Autodesk Inventor part; units mm, degrees
ref_plane "YZ Plane" through (0, 0, 0) normal (1, 0, 0) x (0, 1, 0)
ref_plane "XZ Plane" through (0, 0, 0) normal (0, 1, 0) x (-1, 0, 0)
ref_plane "XY Plane" through (0, 0, 0) normal (0, 0, 1) x (1, 0, 0)
sketch "Skizze1" plane through (0, 0, 0) normal (0, 0, 1) x (1, 0, 0)
  line L0 (-71.4, 0) -> (71.4, 0)
  line L1 (0, -4.2) -> (0, 4.2)
  line L2 (-51, -3) -> (51, -3)
  line L3 (51, -3) -> (51, 3)
  line L4 (51, 3) -> (-51, 3)
  line L5 (-51, 3) -> (-51, -3)
  line L6 (-51, -3) -> (51, 3) construction
  line L7 (51, -3) -> (-51, 3) construction
  point P0 (0, 0)
  dimension "d0" = 102
  dimension "d1" = 6
extrude "Extrusion1" add sketch "Skizze1" against normal blind 348
sketch "Skizze2" plane through (-51, 3, 0) normal (0, 1, 0) x (1, 0, 0)
  line L0 (102, 0) -> (0, 0)
  line L1 (102, 0) -> (102, 348)
  line L2 (0, 348) -> (102, 348)
  line L3 (0, 0) -> (0, 348)
  line L4 (-20.4, 0) -> (122.4, 0)
  line L5 (51, 417.6) -> (51, -69.6)
  line L6 (0, 0) -> (102, 0)
  line L7 (0, 0) -> (6, 0)
  line L8 (6, 0) -> (6, 7)
  line L9 (6, 7) -> (0, 7)
  line L10 (0, 7) -> (0, 0)
  line L11 (102, 0) -> (96, 0)
  line L12 (96, 0) -> (96, 7)
  line L13 (96, 7) -> (102, 7)
  line L14 (102, 7) -> (102, 0)
  line L15 (102, 0) -> (102, 348)
  line L16 (102, 348) -> (96, 348)
  line L17 (96, 348) -> (96, 341)
  line L18 (96, 341) -> (102, 341)
  line L19 (102, 341) -> (102, 348)
  line L20 (102, 348) -> (0, 348)
  line L21 (0, 348) -> (6, 348)
  line L22 (6, 348) -> (6, 341)
  line L23 (6, 341) -> (0, 341)
  line L24 (0, 341) -> (0, 348)
  point P0 (51, 0)
  point P1 (0, 7)
  point P2 (6, 0)
  dimension "d4" = 6
  dimension "d5" = 7
  dimension "d6" = 6
  dimension "d7" = 7
  dimension "d8" = 6
extrude "Extrusion2" cut sketch "Skizze2" against normal blind 348 contours L0 L12 L13 L1 | L18 L17 L2 L1 | L0 L3 L9 L8 | L22 L23 L3 L2
sketch "Skizze3" plane through (51, 3, -7) normal (1, 0, 0) x (0, 0, -1)
  line L0 (334, -6) -> (334, 0)
  line L1 (0, 0) -> (334, 0)
  line L2 (0, 0) -> (0, -6)
  line L3 (0, -6) -> (334, -6)
  point P0 (-7, -3)
  point P1 (23.5, -3)
  point P2 (167, -3)
  point P3 (310.5, -3)
  dimension "d11" = 23.5
  dimension "d12" = 23.5
  dimension "d13" = 167
hole "Bohrung1" at (51, 0, -30.5) at (51, 0, -174) at (51, 0, -317.5) direction (-1, 0, 0) diameter 2.459 depth 8.8 tip angle 118
sketch "Skizze4" plane through (0, 0, 0) normal (0, 0, 1) x (1, 0, 0)
  line L0 (-45, 3) -> (-45, -3)
  line L1 (-45, -3) -> (45, -3)
  line L2 (45, -3) -> (45, 3)
  line L3 (45, 3) -> (-45, 3)
  line L4 (-71.4, 0) -> (71.4, 0)
  line L5 (0, -4.2) -> (0, 4.2)
  point P0 (0, 0)
  point P1 (0, 0)
hole "Bohrung2" at (0, 0, 0) direction (0, 0, -1) diameter 2.459 depth 17 tip angle 118
sketch "Skizze5" plane through (-51, 3, -341) normal (-1, 0, 0) x (0, 0, 1)
  line L0 (334, -6) -> (334, 0)
  line L1 (334, 0) -> (0, 0)
  line L2 (0, 0) -> (0, -6)
  line L3 (334, -6) -> (0, -6)
  circle A0 centre (310.5, -3) radius 1.2295
  circle A1 centre (167, -3) radius 1.2295
  circle A2 centre (23.5, -3) radius 1.2295
  line L4 (341, -7.2) -> (341, 1.2)
  line L5 (-76.6, -3) -> (410.6, -3)
  circle A3 centre (23.5, -3) radius 1.2295
  point P0 (341, -3)
hole "Bohrung3" at (-51, 0, -317.5) at (-51, 0, -174) at (-51, 0, -30.5) direction (1, 0, 0) diameter 2.459 depth 17 tip angle 118
properties part number "I Bodenplatte" material "PVC, hart"
Verification items for the finished model (mm, model axes). A direction names the side the tool comes from. Give positions to 0.01 mm unless a question says otherwise; leave off trailing zeros.
(1) Gauge pin test, flat ends, axial feed: pin 1 (2 mm diameter, centred on y = 0, z = -30.5, fed in from +X); pin 2 (1.8 mm diameter, centred on x = 47, y = -0.5, fed in from +Z); pin 3 (1.8 mm diameter, centred on x = -47, y = 0.5, fed in from -Z). Record the tip position at first contact, or that the pin passes through.
(2) Access from +Z, -Z, +X, -X, +Y, -Y to the whole of each face (thin tool, end or side, straight path). Record for faces 1 (the face through (-48, 0, -341)), 2 (the face through (48, 0, -341)), 3 (the face through (51, 0, -172)), 4 (the face through (-45, 0, -3)), 5 (the face through (45, 0, -3)).
(3) Material ranges on line 1 (Z direction, x = -44.25, y = 0); line 2 (Z direction, x = 48, y = 0); line 3 (X direction, y = 0, z = -13.25), recorded low to high.
Worked out:
1. pin 1: stops at x = 42.06
1. pin 2: stops at z = -7
1. pin 3: stops at z = -341
2. face 1: -Z, -X, +Y, -Y
2. face 2: -Z, +X, +Y, -Y
2. face 3: +Z, -Z, +X, +Y, -Y
2. face 4: +Z, -X, +Y, -Y
2. face 5: +Z, +X, +Y, -Y
3. line 1: z = -348 to -318.73, -316.27 to -175.23, -172.77 to -31.73, -29.27 to 0
3. line 2: z = -341 to -318.73, -316.27 to -175.23, -172.77 to -31.73, -29.27 to -7
3. line 3: x = -51 to -1.23, 1.23 to 51
